Design review of the part built by this model. Coordinates are the model's own, in mm. Coordinates: 2 decimals unless noted, no trailing zeros. Loops run counter-clockwise (first coordinate to the right, second up) from the corner with the lowest first, then second, coordinate; pieces in that order, holes last. Notation, with made-up numbers: (-31, 59) -> (22, 59) arc R32 ccw to (22, 89) -> close; hole circle Ø4 at (-40, 19.25). An arc over 180 degrees is marked (long way). Answer in a Markdown table with one row per item.
Autodesk Inventor part; units mm, degrees
ref_plane "YZ Plane" through (0, 0, 0) normal (1, 0, 0) x (0, 1, 0)
ref_plane "XZ Plane" through (0, 0, 0) normal (0, 1, 0) x (-1, 0, 0)
ref_plane "XY Plane" through (0, 0, 0) normal (0, 0, 1) x (1, 0, 0)
sketch "Sketch1" plane through (0, 0, 0) normal (0, 0, 1) x (1, 0, 0)
  line L0 (-110, -20.8494) -> (-110, 0)
  line L1 (-110, 0) -> (0, 0)
  line L2 (0, 0) -> (0, -105)
  line L3 (0, -105) -> (-39.3892, -105)
  line L4 (-110, -20.8494) -> (-119.38, 0) construction
  line L5 (-119.38, 0) -> (-110, 0) construction
  line L6 (-50.8, -25.4) -> (0, -25.4) construction
  line L7 (0, -25.4) -> (0, 0) construction
  line L8 (0, 0) -> (-50.8, 0) construction
  line L9 (-50.8, 0) -> (-50.8, -25.4) construction
  line L10 (-50.8, -25.4) -> (0, 0) construction
  line L11 (0, -25.4) -> (-50.8, 0) construction
  circle A0 centre (-12.7, -12.7) radius 3
  circle A1 centre (-38.1, -12.7) radius 3
  circle A2 centre (-25.4, -75) radius 15.875
  circle A3 centre (-25.4, -75) radius 30
  line L12 (-50.8, -90.9637) -> (-50.8, -59.0363)
  line L13 (-110, -4.7091) -> (-83.2932, 0)
  arc A4 (-56.3982, -84.7295) -> (-61.7755, -78.3211) centre (-62.3821, -84.2903) ccw
  line L14 (-39.3892, -105) -> (-56.3982, -84.7295)
  arc A5 (-85.9963, -49.4559) -> (-100.0831, -32.6679) centre (-102.5, -49) ccw
  line L15 (-61.7755, -78.3211) -> (-85.9963, -49.4559)
  line L16 (-100.0831, -32.6679) -> (-110, -20.8494)
  circle A6 centre (-95.25, -12.7) radius 3
  circle A7 centre (-57.15, -12.7) radius 3
  point P0 (0, 0)
  point P1 (-25.4, -12.7)
  point P2 (-25.4, -25.4)
  point P3 (-50.8, -75)
  point P4 (0, -90.9637)
  point P5 (-110, -10.4247)
  point P6 (-48.3813, -94.2836)
  point P7 (0, -59.0363)
  point P8 (-25.4, -105)
  dimension "d1" = 119.38
  dimension "d2" = 50.8
  dimension "d3" = 25.4
  dimension "d4" = 25.4
  dimension "d5" = 12.7
  dimension "d6" = 6
  dimension "d7" = 6
  dimension "d11" = 110
  dimension "d12" = 60
  dimension "d13" = 25.4
  dimension "d14" = 25.4
  dimension "d17" = 20.8494
  dimension "d18" = 31.75
  dimension "d21" = 170
  dimension "d22" = 26.7068
  dimension "d24" = 86.6409
  dimension "d25" = 12
  dimension "d26" = 47.6179
  dimension "d28" = 81.3659
  dimension "d29" = 33.02
  dimension "d30" = 49
  dimension "d31" = 50
  dimension "d41" = 19.05
  dimension "d42" = 38.1
extrude "Extrusion1" add sketch "Sketch1" along normal blind 15.4305 contours L0 L13 L1 L2 A3 L14 A4 L15 A5 L16 | L2 A3 L12 | L12 A3
fillet "Fillet1" radius 6 8 edges at (0, -90.9637, 7.7153) (-110, -20.8494, 7.7153) (-110, -4.7091, 7.7153) (-83.2932, 0, 7.7153) (-56.3982, -84.7295, 7.7153) (-61.7755, -78.3211, 7.7153) (-85.9963, -49.4559, 7.7153) (-100.0831, -32.6679, 7.7153)
sketch "Sketch2" plane through (0, 0, 0) normal (0, 0, -1) x (-1, 0, 0)
  circle A0 centre (25.4, -75) radius 15.875
  circle A1 centre (25.4, -75) radius 25.4
  line L0 (7.4395, -92.9605) -> (7.4395, -57.0395)
  line L1 (43.3605, -57.0395) -> (43.3605, -92.9605)
  line L2 (7.4395, -92.9605) -> (25.4, -75)
  line L3 (25.4, -75) -> (43.3605, -57.0395)
  point P0 (0, 0)
  point P1 (25.4, -100.4)
  point P2 (25.4, -49.6)
  dimension "d32" = 50.8
  dimension "d33" = 45
hole "Hole1" at (-7.4395, -92.9605, 0) at (-7.4395, -57.0395, 0) at (-43.3605, -57.0395, 0) at (-43.3605, -92.9605, 0) at (-25.4, -100.4, 0) at (-25.4, -49.6, 0) direction (0, 0, 1) diameter 5.105 end through all
equation "\"d7\" = d6"
properties part number "OUTSIDE_INTAKE_SPACERS" material "3D Print Material - chopped carbon Nylon12 (preferred)"
(1) For pin 1 (2 mm diameter, centred on y = -79.5, z = 12, fed in from +X); pin 2 (5 mm diameter, centred on x = -18.5, z = 7.5, fed in from -Y); pin 3 (1.5 mm diameter, centred on x = -89, z = 13, fed in from +Y), all flat-tipped, find the tip position at first contact; note any pin that passes through.
Evaluation:
| item | result |
|---|---|
| pin 1 | stops at x = 0 |
| pin 2 | stops at y = -104.68 |
| pin 3 | stops at y = -0.87 |
(2) Take a section at A-A on y = -12.7. Give the boundary of the cut face in (x, z).
Evaluation:
| item | result |
|---|---|
| outline | (-110, 0) -> (-98.25, 0) -> (-98.25, 15.43) -> (-110, 15.43) -> close; (-92.25, 0) -> (-60.15, 0) -> (-60.15, 15.43) -> (-92.25, 15.43) -> close; (-54.15, 0) -> (-41.1, 0) -> (-41.1, 15.43) -> (-54.15, 15.43) -> close; (-35.1, 0) -> (-15.7, 0) -> (-15.7, 15.43) -> (-35.1, 15.43) -> close; (-9.7, 0) -> (0, 0) -> (0, 15.43) -> (-9.7, 15.43) -> close |
(3) To check wall thickness, follow probe 1 along Y at (x, z) = (-25.4, 5.25) (1 decimal); probe 2 along X at (y, z) = (-55, 4.75); probe 3 along Y at (x, z) = (-95.25, 11.25). State the ranges of each line that lie inside material, in increasing order.
Evaluation:
| item | result |
|---|---|
| probe 1 | y = -105 to -103, -97.8 to -90.9, -59.1 to -52.2, -47 to 0 |
| probe 2 | x = -81.34 to -44.9, -41.83 to -8.97, -5.9 to 0 |
| probe 3 | y = -34.17 to -15.7, -9.7 to -2.11 |
(4) Draft analysis for pull direction Y (two halves, no side actions). For faces 1 (the cylindrical face through (-108.558, -5.842, 7.823)), 2 (the flat face through (-51.709, -90.318, 7.607)), 3 (the cylindrical face through (-9.84, -13.6, 7.61)), 4 (the cylindrical face through (-8.206, -90.526, 7.823)), state which applies: pulls with the +Y half, pulls with the -Y half, needs draft (parallel to the pull), parting line crosses it, or undercut.
Evaluation:
| item | result |
|---|---|
| face 1 | pulls with the +Y half |
| face 2 | pulls with the -Y half |
| face 3 | undercut |
| face 4 | undercut |
(5) Take a section at D-D on x = -12.7. Give the boundary of the cut face in (y, z) (1 decimal), and give its area (3 significant figures).
Evaluation:
| item | result |
|---|---|
| outline | (-102.2, 0) -> (-84.5, 0) -> (-84.5, 15.4) -> (-102.2, 15.4) -> close; (-65.5, 0) -> (-15.7, 0) -> (-15.7, 15.4) -> (-65.5, 15.4) -> close; (-9.7, 0) -> (0, 0) -> (0, 15.4) -> (-9.7, 15.4) -> close |
| area | 1,190 mm² |
(6) Take a section at B-B on x = -25.4. Give the boundary of the cut face in (y, z) (1 decimal).
Evaluation:
| item | result |
|---|---|
| outline | (-105, 0) -> (-103, 0) -> (-103, 15.4) -> (-105, 15.4) -> close; (-97.8, 0) -> (-90.9, 0) -> (-90.9, 15.4) -> (-97.8, 15.4) -> close; (-59.1, 0) -> (-52.2, 0) -> (-52.2, 15.4) -> (-59.1, 15.4) -> close; (-47, 0) -> (0, 0) -> (0, 15.4) -> (-47, 15.4) -> close |
(7) Take a section at C-C on y = -100.4. Give the boundary of the cut face in (x, z).
Evaluation:
| item | result |
|---|---|
| outline | (-41.36, 0) -> (-27.95, 0) -> (-27.95, 15.43) -> (-41.36, 15.43) -> close; (-22.85, 0) -> (-9.44, 0) -> (-9.44, 15.43) -> (-22.85, 15.43) -> close |
